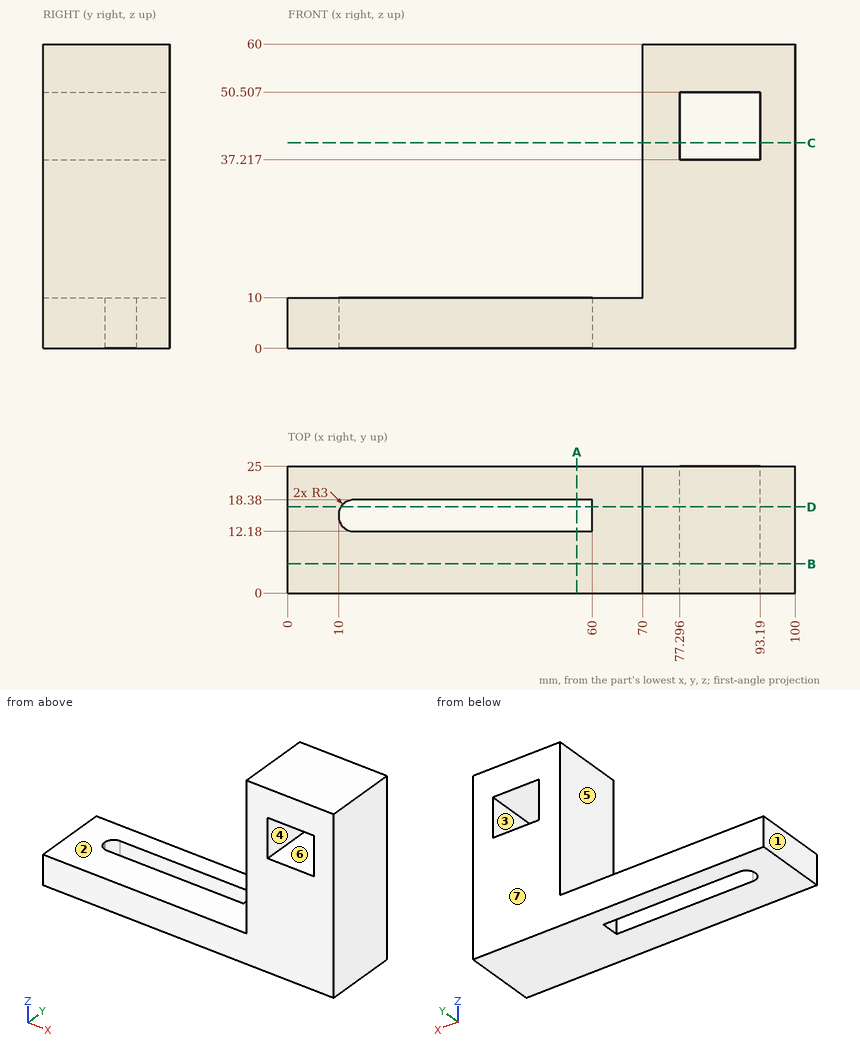
Geometry: see drawing. Coordinates: mm, zero at the bounding-box minimum. A direction names the side the tool comes from. Coordinates: 2 decimals unless noted, no trailing zeros. Loops run counter-clockwise (first coordinate to the right, second up) from the corner with the lowest first, then second, coordinate; pieces in that order, holes last. Notation, with made-up numbers: (-5.5, 23) -> (52.5, 23) arc R9 ccw to (52.5, 32) -> close; hole circle Ø11 at (75.5, 75.25). An arc over 180 degrees is marked (long way). Use a Markdown table: item, result.
1) Cut plane C-C (z = 40.5). Return the cut outline in (x, y).
Results found:
| item | result |
|---|---|
| outline | (70, 0) -> (77.3, 0) -> (77.3, 25) -> (70, 25) -> close; (93.19, 0) -> (100, 0) -> (100, 25) -> (93.19, 25) -> close |
2) Cut plane D-D (y = 17). Return the cut outline in (x, z) (1 decimal), then the cut area to 3 significant figures.
Results found:
| item | result |
|---|---|
| outline | (0, 0) -> (10.5, 0) -> (10.5, 10) -> (0, 10) -> close; (60, 0) -> (100, 0) -> (100, 60) -> (70, 60) -> (70, 10) -> (60, 10) -> close; hole (77.3, 37.2) -> (93.2, 37.2) -> (93.2, 50.5) -> (77.3, 50.5) -> close |
| area | 1,790 mm2 |
3) Contact query for flat-ended pins moving along their axis: pin 1 (1 mm diameter, centred on y = 8, z = 17, fed in from -X); pin 2 (7.5 mm diameter, centred on x = 26.5, y = 7.5, fed in from +Z). Output: stop coordinate, or through.
Results found:
| item | result |
|---|---|
| pin 1 | stops at x = 70 |
| pin 2 | stops at z = 10 |
4) Cut plane A-A (x = 57). Return the cut outline in (y, z), then the cut area to 3 significant figures.
Results found:
| item | result |
|---|---|
| outline | (0, 0) -> (12.18, 0) -> (12.18, 10) -> (0, 10) -> close; (18.38, 0) -> (25, 0) -> (25, 10) -> (18.38, 10) -> close |
| area | 188 mm2 |
5) Cut plane B-B (y = 5.75). Return the cut outline in (x, z).
Results found:
| item | result |
|---|---|
| outline | (0, 0) -> (100, 0) -> (100, 60) -> (70, 60) -> (70, 10) -> (0, 10) -> close; hole (77.3, 37.22) -> (93.19, 37.22) -> (93.19, 50.51) -> (77.3, 50.51) -> close |
6) Access query for the marked faces 1, 2 and 3. Directions: +Z, -Z, +X, -X, +Y, -Y. A direction counts if a zero-diameter tool reaches every point of the face in a straight line with its end or side. Return the directions, or none.
Results found:
| item | result |
|---|---|
| face 1 | +Z, -Z, -X, +Y, -Y |
| face 2 | +Z, -X, +Y, -Y |
| face 3 | +Y, -Y |
7) Material intervals for line 1 along X through (y, z) = (8.25, 45); line 2 along Z through (x, y) = (85.5, 21); line 3 along Y through (x, z) = (46, 8), sorted ascending. Write a range as from..to.
Results found:
| item | result |
|---|---|
| line 1 | x = 70..77.3, 93.19..100 |
| line 2 | z = 0..37.22, 50.51..60 |
| line 3 | y = 0..12.18, 18.38..25 |
8) Pull-direction query (X, two-part tool) for the marked faces 4, 5, 6 and 7; classes: released by +X, released by -X, zero draft, split by the parting line, or undercut.
Results found:
| item | result |
|---|---|
| face 4 | undercut |
| face 5 | released by -X |
| face 6 | undercut |
| face 7 | zero draft |
